CAD build for the part. Positions are in the model's coordinates, mm. Coordinates: 2 decimals unless noted, no trailing zeros. Order: outer loops, then holes, each group sorted by start corner. A loop starts at its lowest first (then second) coordinate and runs counter-clockwise, first axis right, second up. Notation, with made-up numbers: (27.5, -11.5) - (52.5, -11.5) arc R17 ccw to (52.5, 13.5) - close; hole circle Ø9 at (72.5, -8.75). An arc over 180 degrees is marked (long way). Use one line per item in the form item = value.
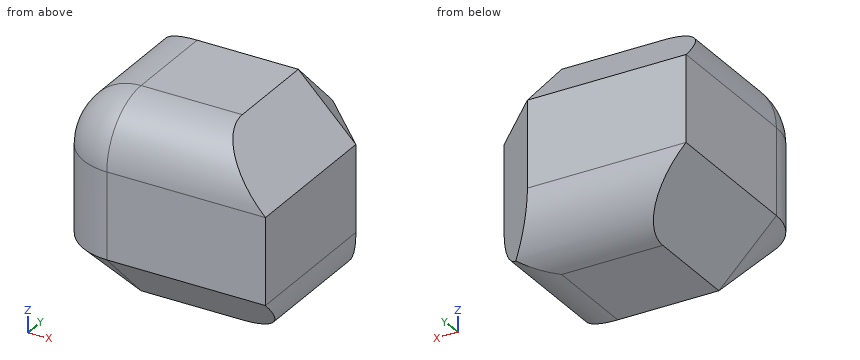
```python
from build123d import *

# Parameters (mm, degrees)
F0_W         = 75.1911774278
F0_H         = 72.7032572031
F1_DEPTH     = 70
F2_R         = 20
F3_T1_DEPTH  = 25.4034118443
F3_T3_DEPTH  = 155.5705767217
F3_T5_DEPTH  = 158.0584969464
F3_T7_DEPTH  = 152.8673195186
F3_T9_DEPTH  = 86.6248371871
F3_T11_DEPTH = 84.1369169624
F3_T14_ANGLE = 90


# Not quite as in the source:
# - a fillet or chamfer that OpenCascade refuses, or shapes differently, is made with other operations: its cross-section is extruded or revolved along the edge and cut away or added


with BuildPart() as f1:
    # F0 (on Top) → F1 (new body)
    with BuildSketch(Plane.XY):
        Rectangle(F0_W, F0_H)
    extrude(amount=F1_DEPTH)

    # F2
    f2_edges = [f1.edges().sort_by_distance(p)[0] for p in [
        (-37.595589, 0, 70),
        (0, -36.351629, 70),
        (-37.595589, -36.351629, 35),
        (0, 36.351629, 0),
        (37.595589, 0, 0),
    ]]
    fillet(f2_edges, radius=F2_R)

    # F3: chamfer of 20 on 6 edges, made by hand

    # F3_s2 → F3_t1 (cut)
    with BuildSketch(Plane(origin=(34.6490724385, 34.6490724385, 34.6490724385), x_dir=(-0.7071067812, 0.7071067812, 0), z_dir=(0.5773502692, 0.5773502692, 0.5773502692))):
        Polygon((-15.0217482547, 18.8009698021), (13.2625229928, 18.8009698021), (-0.879612631, 43.2958672299), align=None)
    extrude(amount=F3_T1_DEPTH, mode=Mode.SUBTRACT)

    # F3_s4 → F3_t3 (cut)
    with BuildSketch(Plane.XZ.offset(-87.7852883609)):
        Polygon((37.5955887139, 50), (17.5955887139, 70), (37.5955887139, 70), align=None)
    extrude(amount=F3_T3_DEPTH, mode=Mode.SUBTRACT)

    # F3_s6 → F3_t5 (cut)
    with BuildSketch(Plane.YZ.offset(-69.0292484732)):
        Polygon((36.3516286016, 50), (16.3516286016, 70), (36.3516286016, 70), align=None)
    extrude(amount=F3_T5_DEPTH, mode=Mode.SUBTRACT)

    # F3_s8 → F3_t7 (cut)
    with BuildSketch(Plane.XY.offset(-31.4336597593)):
        Polygon((37.5955887139, 16.3516286016), (17.5955887139, 36.3516286016), (37.5955887139, 36.3516286016), align=None)
    extrude(amount=F3_T7_DEPTH, mode=Mode.SUBTRACT)

    # F3_s10 → F3_t9 (cut)
    with BuildSketch(Plane.YZ.offset(-17.5955887139)):
        Polygon((-36.3516286016, 20), (-16.3516286016, 0), (-36.3516286016, 0), align=None)
    extrude(amount=F3_T9_DEPTH, mode=Mode.SUBTRACT)

    # F3_s12 → F3_t11 (cut)
    with BuildSketch(Plane.XZ.offset(-67.7852883609)):
        Polygon((-17.5955887139, 0), (-37.5955887139, 20), (-37.5955887139, 0), align=None)
    extrude(amount=F3_T11_DEPTH, mode=Mode.SUBTRACT)

    # F3_s13 → F3_t14 (revolve, cut)
    with BuildSketch(Plane.XZ.offset(16.3516286016)):
        Polygon((-17.5955887139, 0), (-37.5955887139, 20), (-37.5955887139, 0), align=None)
    revolve(axis=Axis((-17.5955887139, -16.3516286016, 0), (0, 0, 1)), revolution_arc=F3_T14_ANGLE, mode=Mode.SUBTRACT)


solid = f1.part
```
Item 1: Cut at B-B, the plane x = -9. Write the cut outline in (y, z).
Derived:
outline = (-36.35, 20) - (-16.35, 0) - (16.35, 0) arc R20 ccw to (36.35, 20) - (36.35, 50) - (16.35, 70) - (-16.35, 70) arc R20 ccw to (-36.35, 50) - close
Item 2: Drop flat-ended pins along their axis: pin 1 (10 mm diameter, centred on x = -10, y = 26, fed in from +Z); pin 2 (1.5 mm diameter, centred on x = 21.5, z = 51.5, fed in from +Y); pin 3 (4 mm diameter, centred on x = -25, y = -10.5, fed in from -Z). Give the stop position or say it passes through.
Derived:
pin_1 = 65.35
pin_2 = 32.01
pin_3 = 5.4
Item 3: Cut at C-C, the plane z = 35.5. Write the cut outline in (x, y).
Derived:
outline = (-37.6, -16.35) arc R20 ccw to (-17.6, -36.35) - (37.6, -36.35) - (37.6, 16.35) - (17.6, 36.35) - (-37.6, 36.35) - close
Item 4: Drill centre lines: line 1 (Z direction, x = 14, y = -18.5); line 2 (Y direction, x = 22.5, z = 14); line 3 (Z direction, x = 21, y = 1.5). Where is each one in solid material? Low to high. Write a range as [from, to].
Derived:
line_1 = [2.15, 69.88]
line_2 = [-30.35, 31.45]
line_3 = [0.29, 66.6]
Item 5: Cut at A-A, the plane y = -3.5. Write the cut outline in (x, z).
Derived:
outline = (-37.6, 20) - (-17.6, 0) - (17.6, 0) arc R20 ccw to (37.6, 20) - (37.6, 50) - (17.6, 70) - (-17.6, 70) arc R20 ccw to (-37.6, 50) - close
Item 6: Cut at D-D, the plane z = 59. Write the cut outline in (x, y).
Derived:
outline = (-35.46, -16.35) arc R17.86 ccw to (-17.6, -34.21) - (28.6, -34.21) - (28.6, 16.35) - (17.6, 27.35) - (-35.46, 27.35) - close
